Input: part model. Units: mm. Frame: model coordinates. A direction names the side the tool comes from. Coordinates: 2 decimals unless noted, no trailing zeros. Write each loop counter-clockwise with the first axis right and the second up, starting at its lowest first coordinate (ties: lowest second). Pieces come first, ordered by that corner, then holes. Notation, with made-up numbers: M 24,-31.5 L 75,-31.5 A17 cw 75,-27.5 Z; hole C 39.5,79.5 d2. An arc over 180 degrees is marked long. Answer as a JSON object with one key per item and string values. Group by question number.
from build123d import *

# Parameters (mm, degrees)
SKETCH_1_W      = 10
SKETCH_1_H      = 4
EXTRUDE_1_DEPTH = 1.2
SKETCH_2_W      = 8
SKETCH_2_H      = 2.4
SKETCH_2_W_2    = 6.8
SKETCH_2_H_2    = 1.6
EXTRUDE_2_DEPTH = 5
FILLET_1_R      = 2
FILLET_2_R      = 0.8
FILLET_3_R      = 0.8
FILLET_4_R      = 0.4
FILLET_5_R      = 0.2


with BuildPart() as part:
    # Эскиз1 → Бобышка-Вытянуть1 (new body)
    with BuildSketch(Plane.XY):
        Rectangle(SKETCH_1_W, SKETCH_1_H)
    extrude(amount=EXTRUDE_1_DEPTH)

    # Эскиз2 → Бобышка-Вытянуть2 (add)
    with BuildSketch(Plane.XY.offset(1.2)):
        Rectangle(SKETCH_2_W, SKETCH_2_H)
        Rectangle(SKETCH_2_W_2, SKETCH_2_H_2, mode=Mode.SUBTRACT)
    extrude(amount=EXTRUDE_2_DEPTH)

    # Скругление1
    fillet_1_edges = [part.edges().sort_by_distance(p)[0] for p in [
        (5, 2, 0.6),
        (5, -2, 0.6),
        (-5, -2, 0.6),
        (-5, 2, 0.6),
    ]]
    fillet(fillet_1_edges, radius=FILLET_1_R - 0.0001)  # a hair under: the kernel refuses the full size

    # Скругление2
    fillet_2_edges = [part.edges().sort_by_distance(p)[0] for p in [
        (0, 2, 0),
        (0, -2, 0),
        (-4.414242852, 1.414242852, 0),
        (-4.414242852, -1.414242852, 0),
        (4.414242852, -1.414242852, 0),
        (4.414242852, 1.414242852, 0),
    ]]
    fillet(fillet_2_edges, radius=FILLET_2_R)

    # Скругление3
    fillet_3_edges = [part.edges().sort_by_distance(p)[0] for p in [
        (4, -1.2, 3.7),
        (4, 1.2, 3.7),
        (-4, 1.2, 3.7),
        (-4, -1.2, 3.7),
    ]]
    fillet(fillet_3_edges, radius=FILLET_3_R)

    # Скругление4
    fillet_4_edges = [part.edges().sort_by_distance(p)[0] for p in [
        (3.4, 0.8, 3.7),
        (-3.4, 0.8, 3.7),
        (-3.4, -0.8, 3.7),
        (3.4, -0.8, 3.7),
    ]]
    fillet(fillet_4_edges, radius=FILLET_4_R)

    # Скругление5
    fillet_5_edges = [part.edges().sort_by_distance(p)[0] for p in [
        (-3.4, 0, 6.2),
        (0, -0.8, 6.2),
        (3.4, 0, 6.2),
        (0, 0.8, 6.2),
        (-3.282842712, -0.682842712, 6.2),
        (3.282842712, -0.682842712, 6.2),
        (3.282842712, 0.682842712, 6.2),
        (-3.282842712, 0.682842712, 6.2),
        (0, -1.2, 6.2),
        (-4, 0, 6.2),
        (4, 0, 6.2),
        (0, 1.2, 6.2),
        (-3.765685425, 0.965685425, 6.2),
        (3.765685425, 0.965685425, 6.2),
        (3.765685425, -0.965685425, 6.2),
        (-3.765685425, -0.965685425, 6.2),
    ]]
    fillet(fillet_5_edges, radius=FILLET_5_R - 0.0001)  # a hair under: the kernel refuses the full size


solid = part.part
Q1. Access query for faces 5 (the flat face through (-4, 0, 4)), 6 (the flat face through (-3.4, 0, 4)), 7 (the flat face through (0, 1.2, 4)), 8 (the flat face through (4, 0, 4)). Directions: +Z, -Z, +X, -X, +Y, -Y. A direction counts if a zero-diameter tool reaches every point of the face in a straight line with its end or side. Return the directions, or none.
Q2. Section A-A, the plane z = 5. Return the cut outline in (x, y).
Q3. Pin query (flat end, axial travel): pin 1 Ø1.5 at (x, y) = (2.5, 1.5) entering from -Z; pin 2 Ø1.4 at (x, z) = (-0.5, 4) entering from +Y; pin 3 Ø1 at (y, z) = (0.5, 3) entering from +X; pin 4 Ø2 at (y, z) = (-0.5, 3) entering from -X. Return the tip coordinate at first contact, or that it passes through.
Q4. Line query: line 1 (X direction, y = -0.2, z = 3.25); line 2 (Y direction, x = 0, z = 3.75); line 3 (Z direction, x = -2, y = 0.75). Output: solid intervals per line, ascending. Write a range as from..to.
Q5. Draft query along X for faces 1 (the flat face through (3.4, 0, 4)), 2 (the cylindrical face through (3.77, 0.96, 3.63)), 3 (the flat face through (0, 0.8, 4)), 4 (the flat face through (0, 0, 0)). Return one class per face: released by +X, released by -X, zero draft, split by the parting line, or undercut.
Filled in:
{
 "1": {"face 5": "+Z, -X, +Y, -Y", "face 6": "+Z", "face 7": "+Z, +X, -X, +Y", "face 8": "+Z, +X, +Y, -Y"},
 "2": {"outline": "M -4,-0.4 A0.8 ccw -3.2,-1.2 L 3.2,-1.2 A0.8 ccw 4,-0.4 L 4,0.4 A0.8 ccw 3.2,1.2 L -3.2,1.2 A0.8 ccw -4,0.4 Z; hole M -3.4,-0.4 A0.4 ccw -3,-0.8 L 3,-0.8 A0.4 ccw 3.4,-0.4 L 3.4,0.4 A0.4 ccw 3,0.8 L -3,0.8 A0.4 ccw -3.4,0.4 Z"},
 "3": {"pin 1": "z = 0", "pin 2": "y = 1.2", "pin 3": "x = 4", "pin 4": "x = -4"},
 "4": {"line 1": "-4..-3.4, 3.4..4", "line 2": "-1.2..-0.8, 0.8..1.2", "line 3": "0..1.2"},
 "5": {"face 1": "undercut", "face 2": "released by +X", "face 3": "undercut", "face 4": "zero draft"}
}
